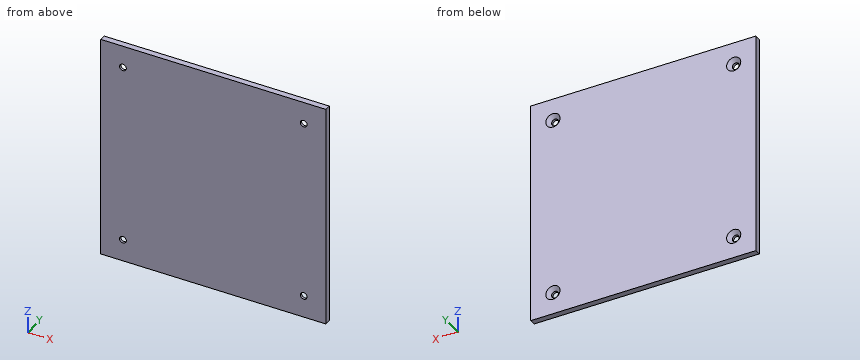
from build123d import *

# Parameters (mm, degrees)
SKETCH1_W                                      = 149.5
SKETCH1_H                                      = 149.5
BASE_FLANGE1_DEPTH                             = 4
CSK_FOR_M4_FLAT_HEAD_MACHINE_SCREW1_AT_2_COUNT = 2
CSK_FOR_M4_FLAT_HEAD_MACHINE_SCREW1_AT_2_PITCH = 120
CSK_FOR_M4_FLAT_HEAD_MACHINE_SCREW1_AT_3_COUNT = 2
CSK_FOR_M4_FLAT_HEAD_MACHINE_SCREW1_AT_3_PITCH = 169.705627485
CSK_FOR_M4_FLAT_HEAD_MACHINE_SCREW1_AT_4_COUNT = 2
CSK_FOR_M4_FLAT_HEAD_MACHINE_SCREW1_AT_4_PITCH = 120


# Sheet-metal steps are written as plain solids
with BuildPart() as part:
    # Sketch1 → Base-Flange1 (new body)
    with BuildSketch(Plane(origin=(0, 0, 0), x_dir=(1, 0, 0), z_dir=(0, 1, 0))):
        Rectangle(SKETCH1_W, SKETCH1_H)
    extrude(amount=-BASE_FLANGE1_DEPTH)

    # Sketch5 → CSK for M4 Flat Head Machine Screw1 (revolve, cut)
    with BuildSketch(Plane(origin=(60, 0, -60), x_dir=(0, 0, 1), z_dir=(1, 0, 0))):
        Polygon((0, 0), (0, 4), (2.25, 4), (2.25, 2.45), (4.7, 0), align=None)
    csk_for_m4_flat_head_machine_screw1 = revolve(axis=Axis((60, 6.35, -60), (0, -1, 0)), mode=Mode.SUBTRACT)

    # CSK for M4 Flat Head Machine Screw1 at 2: CSK for M4 Flat Head Machine Screw1 ×2
    with Locations(*[(-i * CSK_FOR_M4_FLAT_HEAD_MACHINE_SCREW1_AT_2_PITCH, 0, 0) for i in range(1, CSK_FOR_M4_FLAT_HEAD_MACHINE_SCREW1_AT_2_COUNT)]):
        add(csk_for_m4_flat_head_machine_screw1, mode=Mode.SUBTRACT)

    # CSK for M4 Flat Head Machine Screw1 at 3: CSK for M4 Flat Head Machine Screw1 ×2
    with Locations(*[Vector(-0.7071067811865475, 0, 0.7071067811865476) * (i * CSK_FOR_M4_FLAT_HEAD_MACHINE_SCREW1_AT_3_PITCH) for i in range(1, CSK_FOR_M4_FLAT_HEAD_MACHINE_SCREW1_AT_3_COUNT)]):
        add(csk_for_m4_flat_head_machine_screw1, mode=Mode.SUBTRACT)

    # CSK for M4 Flat Head Machine Screw1 at 4: CSK for M4 Flat Head Machine Screw1 ×2
    with Locations(*[(0, 0, i * CSK_FOR_M4_FLAT_HEAD_MACHINE_SCREW1_AT_4_PITCH) for i in range(1, CSK_FOR_M4_FLAT_HEAD_MACHINE_SCREW1_AT_4_COUNT)]):
        add(csk_for_m4_flat_head_machine_screw1, mode=Mode.SUBTRACT)


solid = part.part
Design review of the part built by this model. Coordinates are the model's own, in mm. Round coordinates to 2 decimals unless told otherwise and drop trailing zeros. Write each loop counter-clockwise with the first axis right and the second up, starting at its lowest first coordinate (ties: lowest second). Pieces come first, ordered by that corner, then holes. Notation, with made-up numbers: (83, -37.75) - (138, -37.75) arc R13 ccw to (138, -14.75) - close; hole circle Ø5 at (81, -11). An arc over 180 degrees is marked (long way). Use a Markdown table: item, result. Add a question column.
1. We need section A-A (x = -60). State the section outline as (y, z) points, then the cut area to 3 significant figures.
2. Clearance check with flat-ended pins moving along their axes: pin 1 (3.5 mm diameter, centred on x = -60, z = -60, fed in from -Y); pin 2 (5 mm diameter, centred on x = 60, z = 60, fed in from +Y). State where each tip first meets the part, or that it passes through.
3. We need section B-B (z = -60). State the section outline as (x, y) points, then the cut area to 3 significant figures.
4. Wall thickness on probe 1 along X at (y, z) = (-3.55, -60): over which ranges is the line inside the solid? List them lowest first.
Output:
| question | item | result |
|---|---|---|
| 1 | outline | (-4, -74.75) - (0, -74.75) - (0, -64.7) - (-2.45, -62.25) - (-4, -62.25) - close; (-4, -57.75) - (-2.45, -57.75) - (0, -55.3) - (0, 55.3) - (-2.45, 57.75) - (-4, 57.75) - close; (-4, 62.25) - (-2.45, 62.25) - (0, 64.7) - (0, 74.75) - (-4, 74.75) - close |
| 1 | area | 550 mm2 |
| 2 | pin 1 | passes through |
| 2 | pin 2 | stops at y = -2.2 |
| 3 | outline | (-74.75, -4) - (-62.25, -4) - (-62.25, -2.45) - (-64.7, 0) - (-74.75, 0) - close; (-57.75, -4) - (57.75, -4) - (57.75, -2.45) - (55.3, 0) - (-55.3, 0) - (-57.75, -2.45) - close; (62.25, -4) - (74.75, -4) - (74.75, 0) - (64.7, 0) - (62.25, -2.45) - close |
| 3 | area | 550 mm2 |
| 4 | probe 1 | x = -74.75 to -62.25, -57.75 to 57.75, 62.25 to 74.75 |
